Check sheet for the modelled part. Datum: model origin and axes. Units: mm. Face numbers are marked on the shaded views. A direction names the side the tool comes from. Round coordinates to 2 decimals unless told otherwise and drop trailing zeros. Order: outer loops, then holes, each group sorted by start corner. A loop starts at its lowest first (then second) coordinate and runs counter-clockwise, first axis right, second up. Notation, with made-up numbers: (-1, 62) -> (50, 62) arc R21 cw to (50, 93) -> close; hole circle Ø10 at (10.25, 57). An arc over 180 degrees is marked (long way). Answer in a Markdown table with one row per item.
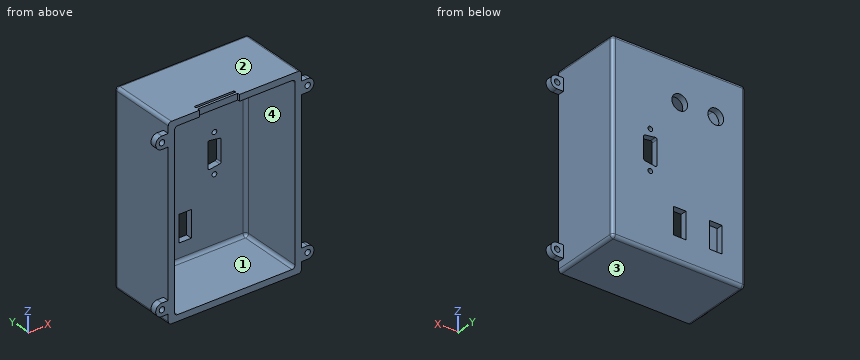
```python
from build123d import *

# Parameters (mm, degrees)
SKETCH1_W               = 85
SKETCH1_H               = 120
BOSS_EXTRUDE1_DEPTH     = 20
SHELL2_T                = -4
SKETCH4_R               = 5
SKETCH4_W               = 8
SKETCH4_H               = 17
CUT_EXTRUDE1_DEPTH      = 20
SKETCH5_W               = 25.5
SKETCH5_H               = 1.5
CUT_EXTRUDE2_DEPTH      = 20
SKETCH6_R               = 1.75
BOSS_EXTRUDE2_DEPTH     = 4
CUT_EXTRUDE3_DEPTH      = 159.347718645
CUT_EXTRUDE3_DEPTH_BACK = 10
SKETCH7_W               = 25.5
SKETCH7_H               = 1.512902769
CUT_EXTRUDE4_START      = 45
SKETCH8_R               = 1.5
CUT_EXTRUDE4_DEPTH      = 10
FILLET1_R               = 1
FILLET2_R               = 2
FILLET3_R               = 2


with BuildPart() as part:
    # Sketch1 → Boss-Extrude1 (new body)
    with BuildSketch(Plane(origin=(0, 0, 0), x_dir=(1, 0, 0), z_dir=(0, 1, 0))):
        with Locations((42.5, 60)):
            Rectangle(SKETCH1_W, SKETCH1_H)
    extrude(amount=BOSS_EXTRUDE1_DEPTH)

    # Sketch2 → section 0 of loft1
    with BuildSketch(Plane(origin=(0, 45, 0), x_dir=(1, 0, 0), z_dir=(0, 1, 0)), mode=Mode.PRIVATE) as loft1_s0:
        with BuildLine():
            Line((0, 120), (85, 120))
            Line((85, 120), (85, 0))
            Line((85, 0), (0, 0))
            Line((0, 0), (0, 120))
        make_face()
    # loft up to a face of the part (loft1)
    loft([loft1_s0.sketch, part.faces().sort_by_distance((42.5, 20, -60))[0]])

    # Shell2
    shell2_openings = [part.faces().sort_by_distance(p)[0] for p in [
        (42.5, 0, -60),
    ]]
    offset(amount=SHELL2_T, openings=shell2_openings, kind=Kind.INTERSECTION)

    # Sketch4 → Cut-Extrude1 (cut)
    with BuildSketch(Plane(origin=(0, 45, 0), x_dir=(1, 0, 0), z_dir=(0, 1, 0))):
        with Locations(Location((19, 25, 0), (0, 0, 270))):
            Circle(SKETCH4_R)
        with Locations(Location((42, 25, 0), (0, 0, 270))):
            Circle(SKETCH4_R)
        with Locations((19, 96.5)):
            Rectangle(SKETCH4_W, SKETCH4_H)
        with Locations((42, 96.5)):
            Rectangle(SKETCH4_W, SKETCH4_H)
    extrude(amount=-CUT_EXTRUDE1_DEPTH, mode=Mode.SUBTRACT)

    # Sketch5 → Cut-Extrude2 (cut)
    with BuildSketch(Plane.XY):
        with Locations((32.75, 0.75)):
            Rectangle(SKETCH5_W, SKETCH5_H)
    extrude(amount=-CUT_EXTRUDE2_DEPTH, mode=Mode.SUBTRACT)

    # Sketch6 → Boss-Extrude2 (add)
    # profile 1 of 4: a face of its own
    with BuildSketch(Plane(origin=(0, 0, 0), x_dir=(-1, 0, 0), z_dir=(0, -1, 0))):
        with BuildLine():
            Line((-85, 6.5), (-89, 6.5))
            ThreePointArc((-89, 6.5), (-93, 10.5), (-89, 14.5))
            Line((-89, 14.5), (-85, 14.5))
            Line((-85, 14.5), (-85, 6.5))
        make_face()
        with Locations(Location((-89, 10.5, 0), (0, 0, 90))):
            Circle(SKETCH6_R, mode=Mode.SUBTRACT)
    # profile 2 of 4: a face of its own
    with BuildSketch(Plane(origin=(0, 0, 0), x_dir=(-1, 0, 0), z_dir=(0, -1, 0))):
        with BuildLine():
            Line((-85, 113.5), (-89, 113.5))
            ThreePointArc((-89, 113.5), (-93, 109.5), (-89, 105.5))
            Line((-89, 105.5), (-85, 105.5))
            Line((-85, 105.5), (-85, 113.5))
        make_face()
        with Locations(Location((-89, 109.5, 0), (0, 0, 90))):
            Circle(SKETCH6_R, mode=Mode.SUBTRACT)
    # profile 3 of 4: a face of its own
    with BuildSketch(Plane(origin=(0, 0, 0), x_dir=(-1, 0, 0), z_dir=(0, -1, 0))):
        with BuildLine():
            Line((0, 113.5), (4, 113.5))
            ThreePointArc((4, 113.5), (8, 109.5), (4, 105.5))
            Line((4, 105.5), (0, 105.5))
            Line((0, 105.5), (0, 113.5))
        make_face()
        with Locations(Location((4, 109.5, 0), (0, 0, 90))):
            Circle(SKETCH6_R, mode=Mode.SUBTRACT)
    # profile 4 of 4: a face of its own
    with BuildSketch(Plane(origin=(0, 0, 0), x_dir=(-1, 0, 0), z_dir=(0, -1, 0))):
        with BuildLine():
            Line((0, 14.5), (4, 14.5))
            ThreePointArc((4, 14.5), (8, 10.5), (4, 6.5))
            Line((4, 6.5), (0, 6.5))
            Line((0, 6.5), (0, 14.5))
        make_face()
        with Locations(Location((4, 10.5, 0), (0, 0, 90))):
            Circle(SKETCH6_R, mode=Mode.SUBTRACT)
    extrude(amount=-BOSS_EXTRUDE2_DEPTH)

    # Sketch7 → Cut-Extrude3 (cut, two sides: drawn at the far end of the back side and taken through both)
    with BuildSketch(Plane.XY.offset(-CUT_EXTRUDE3_DEPTH_BACK)):
        with Locations((32.75, 3.769108467)):
            Rectangle(SKETCH7_W, SKETCH7_H)
    extrude(amount=CUT_EXTRUDE3_DEPTH + CUT_EXTRUDE3_DEPTH_BACK, mode=Mode.SUBTRACT)

    # Sketch8 → Cut-Extrude4 (cut)
    with BuildSketch(Plane(origin=(0, 0, 0), x_dir=(1, 0, 0), z_dir=(0, 1, 0)).offset(CUT_EXTRUDE4_START)):
        with Locations(Location((60.75, 72.5, 0), (0, 0, 270))):
            Circle(SKETCH8_R)
        with Locations(Location((60.75, 47.5, 0), (0, 0, 270))):
            Circle(SKETCH8_R)
        Polygon((56.5, 68.75), (56.5, 51.25), (65, 52.5), (65, 67.5), align=None)
    extrude(amount=-CUT_EXTRUDE4_DEPTH, mode=Mode.SUBTRACT)

    # Fillet1
    fillet1_edges = [part.edges().sort_by_distance(p)[0] for p in [
        (56.5, 43, -51.25),
        (56.5, 43, -68.75),
        (65, 43, -67.5),
        (65, 43, -52.5),
    ]]
    fillet(fillet1_edges, radius=FILLET1_R)

    # Fillet2
    fillet2_edges = [part.edges().sort_by_distance(p)[0] for p in [
        (4, 20.5, -116),
        (4, 20.5, -4),
        (81, 20.5, -4),
        (81, 20.5, -116),
        (4, 41, -60),
        (42.5, 41, -4),
        (81, 41, -60),
        (42.5, 41, -116),
    ]]
    fillet(fillet2_edges, radius=FILLET2_R)

    # Fillet3
    fillet3_edges = [part.edges().sort_by_distance(p)[0] for p in [
        (0, 45, -60),
        (42.5, 45, 0),
        (85, 45, -60),
        (42.5, 45, -120),
        (0, 22.5, -120),
        (85, 22.5, -120),
        (85, 22.5, 0),
        (0, 22.5, 0),
    ]]
    fillet(fillet3_edges, radius=FILLET3_R)


solid = part.part
```
(1) Section check C-C on y = 36.5. Record the boundary of the cut face in (x, z), plus the area to 3 significant figures.
Solutions:
| item | result |
|---|---|
| outline | (0, -118) arc R2 ccw to (2, -120) -> (83, -120) arc R2 ccw to (85, -118) -> (85, -2) arc R2 ccw to (83, 0) -> (2, 0) arc R2 ccw to (0, -2) -> close; hole (4, -114) arc R2 ccw to (6, -116) -> (79, -116) arc R2 ccw to (81, -114) -> (81, -6) arc R2 ccw to (79, -4) -> (6, -4) arc R2 ccw to (4, -6) -> close |
| area | 1,580 mm^2 |
(2) Tool access check on the marked faces 3 and 4. Record the directions out of +Z, -Z, +X, -X, +Y, -Y that give a thin tool (end or side, any length) a straight path to the whole face; none if there is none.
Solutions:
| item | result |
|---|---|
| face 3 | -Z, +X, -X, +Y, -Y |
| face 4 | -Y |
(3) Section check D-D on z = -72.5. Record the boundary of the cut face in (x, y), plus the area to 3 significant figures.
Solutions:
| item | result |
|---|---|
| outline | (0, 0) -> (4, 0) -> (4, 39) arc R2 cw to (6, 41) -> (59.25, 41) -> (59.25, 45) -> (2, 45) arc R2 ccw to (0, 43) -> close; (62.25, 41) -> (79, 41) arc R2 cw to (81, 39) -> (81, 0) -> (85, 0) -> (85, 43) arc R2 ccw to (83, 45) -> (62.25, 45) -> close |
| area | 656 mm^2 |
(4) Depth check by flat-ended pin: pin 1 Ø2 at (x, y) = (-3, 2.5) entering from +Z; pin 2 Ø4.5 at (y, z) = (43, -95) entering from +X; pin 3 Ø9 at (x, z) = (88, -11) entering from +Y. Enter the tip coordinate at first touch or a pass-through.
Solutions:
| item | result |
|---|---|
| pin 1 | z = -6.5 |
| pin 2 | x = 85 |
| pin 3 | y = 44.94 |
(5) Section check A-A on x = 42. Record the boundary of the cut face in (y, z).
Solutions:
| item | result |
|---|---|
| outline | (0, -120) -> (43, -120) arc R2 ccw to (45, -118) -> (45, -105) -> (41, -105) -> (41, -114) arc R2 cw to (39, -116) -> (0, -116) -> close; (1.5, -4) -> (3.01, -4) -> (3.01, 0) -> (1.5, 0) -> close; (4.53, -4) -> (39, -4) arc R2 cw to (41, -6) -> (41, -20) -> (45, -20) -> (45, -2) arc R2 ccw to (43, 0) -> (4.53, 0) -> close; (41, -88) -> (45, -88) -> (45, -30) -> (41, -30) -> close |
(6) Draft check along X on the marked faces 1 and 2. Enter one of: pulls with the +X half, pulls with the -X half, needs draft (parallel to the pull), parting line crosses it, or undercut.
Solutions:
| item | result |
|---|---|
| face 1 | undercut |
| face 2 | needs draft |
(7) Section check B-B on z = -25. Record the boundary of the cut face in (x, y), plus the area to 3 significant figures.
Solutions:
| item | result |
|---|---|
| outline | (0, 0) -> (4, 0) -> (4, 39) arc R2 cw to (6, 41) -> (14, 41) -> (14, 45) -> (2, 45) arc R2 ccw to (0, 43) -> close; (24, 41) -> (37, 41) -> (37, 45) -> (24, 45) -> close; (47, 41) -> (79, 41) arc R2 cw to (81, 39) -> (81, 0) -> (85, 0) -> (85, 43) arc R2 ccw to (83, 45) -> (47, 45) -> close |
| area | 588 mm^2 |
(8) Scan lines: probe 1 along Z at (x, y) = (89, 2); probe 2 along Z at (x, y) = (68, 4.5); probe 3 along X at (y, z) = (25, -24). Record each from-to range of solid material in increasing order. Write a range as from..to.
Solutions:
| item | result |
|---|---|
| probe 1 | -113.5..-111.25, -107.75..-105.5, -14.5..-12.25, -8.75..-6.5 |
| probe 2 | -120..-116, -4..0 |
| probe 3 | 0..4, 81..85 |
